Check sheet for the drawn part. Datum: minimum x, y, z corner. Units: mm. A direction names the side the tool comes from. Coordinates: 2 decimals unless noted, no trailing zeros. Write each loop counter-clockwise with the first axis right and the second up, starting at its lowest first coordinate (ties: lowest second). Pieces come first, ordered by that corner, then holes. Notation, with made-up numbers: M 1,39 L 21,39 A13 cw 21,61 Z; hole C 2.25,-1 d1. An arc over 180 degrees is marked long. Answer as a JSON object with one key per item and string values. Group by question number.
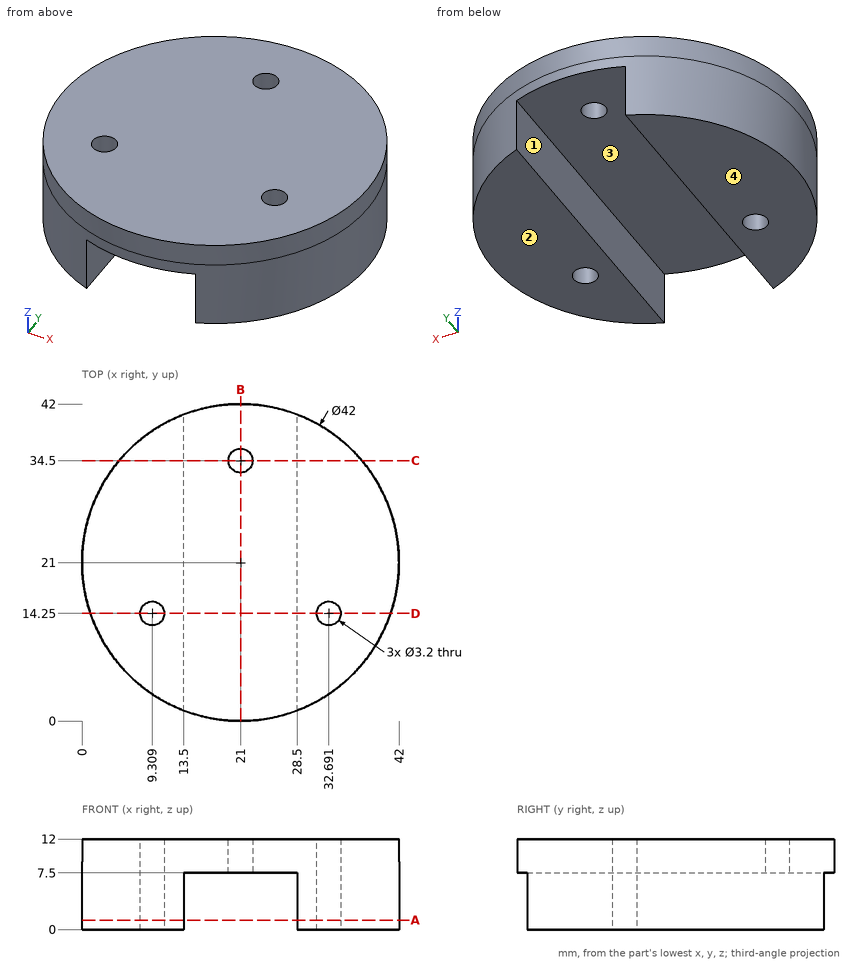
1) Set-up check for the marked faces 1 and 2: record each of +Z, -Z, +X, -X, +Y, -Y from which the full face is reachable in a straight line by a thin tool's end or side.
2) Section check A-A (z = 1.25). State how many separate pieces and enclosed holes the cut face has, then the cut area to 3 significant figures.
3) Go/stop test with flat-tipped pins: pin 1 Ø1 at (x, z) = (9.5, 1.5) entering from +Y; pin 2 Ø2 at (y, z) = (20.5, 3.5) entering from +X; pin 3 Ø4 at (x, z) = (28.5, 9.5) entering from -Y; pin 4 Ø1.5 at (x, z) = (27.5, 9.5) entering from +Y. Record where each tip stops, or that it passes through.
4) Section check B-B (x = 21). Record the cut outline in (y, z).
5) Section check D-D (y = 14.25). Record the cut outline in (x, z) (1 decimal), then the cut area to 3 significant figures.
6) Material ranges on probe 1 along Y at (x, z) = (21, 10.3); probe 2 along Z at (x, y) = (24, 30.5); probe 3 along X at (y, z) = (22.5, 5.25), recorded low to high. Write a range as [from, to].
7) Section check C-C (y = 34.5). Record the cut outline in (x, z), then the cut area to 3 significant figures.
8) Draft check along X on the marked faces 3 and 4. Enter one of: +X half, -X half, draft (parallel to the pull), parting line (faces both ways), or undercut.
Entries:
{
 "1": {"face 1": "-Z, +Y, -Y", "face 2": "-Z, +X, -X, +Y, -Y"},
 "2": {"separate pieces": "2", "enclosed holes": "2", "area": "753 mm^2"},
 "3": {"pin 1": "y = 38.89", "pin 2": "x = 42", "pin 3": "y = 0.73", "pin 4": "y = 41.2"},
 "4": {"outline": "M 0,7.5 L 32.9,7.5 L 32.9,12 L 0,12 Z; M 36.1,7.5 L 42,7.5 L 42,12 L 36.1,12 Z"},
 "5": {"outline": "M 1.1,0 L 7.7,0 L 7.7,12 L 1.1,12 Z; M 10.9,0 L 13.5,0 L 13.5,7.5 L 28.5,7.5 L 28.5,0 L 31.1,0 L 31.1,12 L 10.9,12 Z; M 34.3,0 L 40.9,0 L 40.9,12 L 34.3,12 Z", "area": "288 mm^2"},
 "6": {"probe 1": "[0, 32.9], [36.1, 42]", "probe 2": "[7.5, 12]", "probe 3": "[0.05, 13.5], [28.5, 41.95]"},
 "7": {"outline": "M 4.91,0 L 13.5,0 L 13.5,7.5 L 19.4,7.5 L 19.4,12 L 4.91,12 Z; M 22.6,7.5 L 28.5,7.5 L 28.5,0 L 37.09,0 L 37.09,12 L 22.6,12 Z", "area": "259 mm^2"},
 "8": {"face 3": "undercut", "face 4": "draft"}
}
